Could you check a few things on this model? Use its own coordinates, in mm. A direction names the side the tool comes from. Coordinates: 2 decimals unless noted, no trailing zeros. Order: outer loops, then holes, each group sorted by start corner. A loop starts at its lowest first (then second) coordinate and runs counter-clockwise, first axis right, second up. Notation, with made-up numbers: (31, 64.25) -> (57, 64.25) arc R28 ccw to (57, 94.25) -> close; hole circle Ø11 at (5.25, -31.75). An arc over 180 degrees is marked (long way). Put each result on its own line as item: value. Start each with the question number.
Q1. If we section it at D-D (z = 3.25): Please give me the cut outline in (x, y), and give its area (3 significant figures).
Q2. Please list where these lines run through material, in increasing order: line 1 along Z through (x, y) = (4, -2.85); line 2 along Y through (x, z) = (4, 4); line 3 along Z through (x, y) = (6, -2.9).
Q3. Will this pin go through, and if not, where does the flat tip stop? pin 1 (1.8 mm diameter, centred on x = 7, y = -2.91, fed in from -Z).
Q4. If we section it at A-A (z = 15): Please give me the cut outline in (x, y), and give its area (3 significant figures).
Q5. If we section it at C-C (x = 7): Please give me the cut outline in (y, z).
Q6. For faces 1 (the face through (5, 0, 10)), 2 (the face through (6.76, -3.98, 4.93)), which set-ups out of +Z, -Z, +X, -X, +Y, -Y let a thin tool reach every point of the face, with its end or its side?
Q7. If we section it at B-B (x = 9): Please give me the cut outline in (y, z).
Q8. We'd pull the mould along X, two halves only. Please class faces 3 (the face through (10, -3, 9)), 4 (the face through (0, -3, 9)), 5 (the face through (7, -3, 10)): +X half, -X half, draft (parallel to the pull), parting line (faces both ways), or undercut.
from build123d import *

# Parameters (mm, degrees)
F0_W     = 10
F0_H     = 19
F1_DEPTH = 6
F2_R     = 1.1
F3_DEPTH = 10
F4_R     = 1.1
F5_DEPTH = 10


with BuildPart() as f1:
    # F0 (on Front) → F1 (new body)
    with BuildSketch(Plane.XZ):
        with Locations((5, 9.5)):
            Rectangle(F0_W, F0_H)
    extrude(amount=F1_DEPTH)

    # F2 (on face) → F3 (cut)
    with BuildSketch(Plane.YZ.offset(10)):
        with Locations((-2.874218, 4)):
            Circle(F2_R)
        with Locations((-2.874218, 15)):
            Circle(F2_R)
    extrude(amount=-F3_DEPTH, mode=Mode.SUBTRACT)

    # F4 (on Top) → F5 (cut)
    with BuildSketch(Plane.XY):
        with Locations((7, -2.907384)):
            Circle(F4_R)
    extrude(amount=F5_DEPTH, mode=Mode.SUBTRACT)


solid = f1.part
The answers:
1. outline: (0, -6) -> (10, -6) -> (10, -3.68) -> (7.78, -3.68) arc R1.1 cw to (6.22, -3.68) -> (0, -3.68) -> close; (0, -2.07) -> (6.29, -2.07) arc R1.1 cw to (7.71, -2.07) -> (10, -2.07) -> (10, 0) -> (0, 0) -> close
1. area: 43.3 mm^2
2. line 1: 0 to 2.9, 5.1 to 13.9, 16.1 to 19
2. line 2: -6 to -3.97, -1.77 to 0
2. line 3: 10 to 13.9, 16.1 to 19
3. pin 1: z = 10
4. outline: (0, -6) -> (10, -6) -> (10, -3.97) -> (0, -3.97) -> close; (0, -1.77) -> (10, -1.77) -> (10, 0) -> (0, 0) -> close
4. area: 38.0 mm^2
5. outline: (-6, 0) -> (-4.01, 0) -> (-4.01, 10) -> (-1.81, 10) -> (-1.81, 4.27) arc R1.1 cw to (-1.81, 3.73) -> (-1.81, 0) -> (0, 0) -> (0, 19) -> (-6, 19) -> close; hole circle Ø2.2 at (-2.87, 15)
6. face 1: +Z, -Z, +X, -X, +Y
6. face 2: -Z
7. outline: (-6, 0) -> (0, 0) -> (0, 19) -> (-6, 19) -> close; hole circle Ø2.2 at (-2.87, 4); hole circle Ø2.2 at (-2.87, 15)
8. face 3: +X half
8. face 4: -X half
8. face 5: undercut
